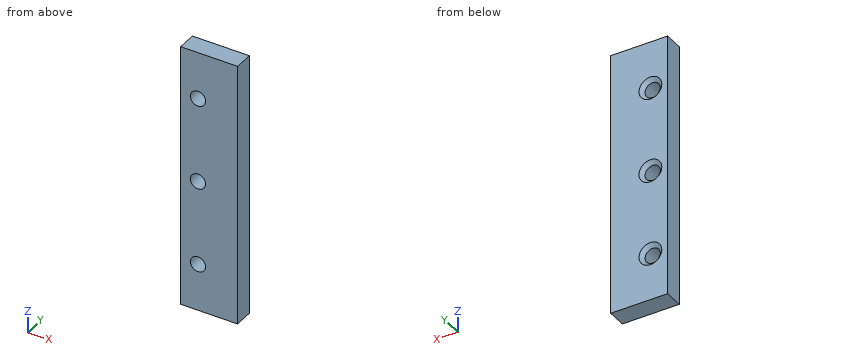
from build123d import *

# Parameters (mm, degrees)
SKETCH1_W                         = 19.05
SKETCH1_H                         = 88.9
BOSS_EXTRUDE1_DEPTH               = 6.35
F_1_4_20_TAPPED_HOLE1_D           = 5.1054
F_1_4_20_TAPPED_HOLE1_CSINK_D     = 7.62
F_1_4_20_TAPPED_HOLE1_CSINK_ANGLE = 90


with BuildPart() as part:
    # Sketch1 → Boss-Extrude1 (new body)
    with BuildSketch(Plane(origin=(0, 0, 0), x_dir=(1, 0, 0), z_dir=(0, 1, 0))):
        with Locations((-9.525, 44.45)):
            Rectangle(SKETCH1_W, SKETCH1_H)
    extrude(amount=BOSS_EXTRUDE1_DEPTH)

    # 1/4-20 Tapped Hole1 (through all)
    with Locations(Plane(origin=(0, 6.35, 0), x_dir=(1, 0, 0), z_dir=(0, 1, 0))):
        with Locations((-13.284419072, 15.875), (-13.284419072, 44.45), (-13.284419072, 73.025)):
            CounterSinkHole(F_1_4_20_TAPPED_HOLE1_D / 2, F_1_4_20_TAPPED_HOLE1_CSINK_D / 2, counter_sink_angle=F_1_4_20_TAPPED_HOLE1_CSINK_ANGLE)


solid = part.part
Build history of the part. All positions in model axes, mm. Coordinates: 2 decimals unless noted, no trailing zeros. Order: outer loops, then holes, each group sorted by start corner. A loop starts at its lowest first (then second) coordinate and runs counter-clockwise, first axis right, second up. Notation, with made-up numbers: (-10, 2) - (28, 2) arc R24 cw to (28, 19) - close; hole circle Ø2 at (-8.5, -37.5). An arc over 180 degrees is marked (long way). Write item = value, one per line. Start each with the question number.
1) Saw through at A-A on z = -44.45. Write the cut outline in (x, y).
2) Flat gauge pin, fed straight in: pin 1 Ø6 at (x, z) = (-13.28, -44.45) entering from +Y. Where does the tip first touch, or does it go through?
3) Wall check: line 1 along Z through (x, y) = (-13.25, 1.25); line 2 along X through (y, z) = (2.55, -44.45); line 3 along Z through (x, y) = (-11, 3.75). Give the ranges that are in metal, low to high. Write a range as from..to.
4) Saw through at B-B on y = 3.5. Write the cut outline in (x, z) (3 decimals), then the cut area to 3 significant figures.
5) Saw through at C-C on x = -12. Count the separate pieces of the cut face and the enclosed holes in it, then the cut area to 3 significant figures.
From the geometry:
q1.outline = (-19.05, 0) - (-15.84, 0) - (-15.84, 5.09) - (-17.09, 6.35) - (-19.05, 6.35) - close; (-10.73, 0) - (0, 0) - (0, 6.35) - (-9.47, 6.35) - (-10.73, 5.09) - close
q2.pin_1 = 5.54
q3.line_1 = -88.9..-75.58, -70.47..-47, -41.9..-18.43, -13.32..0
q3.line_2 = -19.05..-15.84, -10.73..0
q3.line_3 = -88.9..-74.16, -71.89..-45.59, -43.31..-17.01, -14.74..0
q4.outline = (-19.05, -88.9) - (0, -88.9) - (0, 0) - (-19.05, 0) - close; hole circle Ø5.105 at (-13.284, -73.025); hole circle Ø5.105 at (-13.284, -44.45); hole circle Ø5.105 at (-13.284, -15.875)
q4.area = 1,630 mm^2
q5.separate_pieces = 4
q5.enclosed_holes = 0
q5.area = 475 mm^2
